from build123d import *

# Parameters (mm, degrees)
SKETCH1_R           = 3
BOSS_EXTRUDE1_DEPTH = 2.5
SKETCH2_R           = 1.5
BOSS_EXTRUDE2_DEPTH = 20
CHAMFER1_SIZE       = 2.5
CHAMFER1_SIZE_2     = 1.5
FILLET1_R           = 0.1
SKETCH3_W           = 1
SKETCH3_H           = 1
CUT_EXTRUDE2_DEPTH  = 1.5
CHAMFER7_SIZE       = 1.5
CHAMFER7_SIZE_2     = 0.3


with BuildPart() as part:
    # Sketch1 → Boss-Extrude1 (new body)
    with BuildSketch(Plane(origin=(0, 0, 0), x_dir=(1, 0, 0), z_dir=(0, 1, 0))):
        with Locations(Location((0, 0, 0), (0, 0, 270))):
            Circle(SKETCH1_R)
    extrude(amount=BOSS_EXTRUDE1_DEPTH)

    # Sketch2 → Boss-Extrude2 (add)
    with BuildSketch(Plane(origin=(0, 2.5, 0), x_dir=(1, 0, 0), z_dir=(0, 1, 0))):
        with Locations(Location((0, 0, 0), (0, 0, 270))):
            Circle(SKETCH2_R)
    extrude(amount=BOSS_EXTRUDE2_DEPTH)

    # Chamfer1
    # the kernel refuses this chamfer: 2.5, 1.5 mm, written as the material it takes off along each edge
    with BuildSketch(Plane(origin=(0, 2.5, 0), x_dir=(0, 0, 1), z_dir=(-1, 0, 0))) as chamfer1_piece_1_section:
        Polygon((3, -CHAMFER1_SIZE), (3 - CHAMFER1_SIZE_2, 0), (3, 0), align=None)
    chamfer1_piece_1 = revolve(axis=Axis((0, 2.5, 0), (0, 1, 0)), mode=Mode.PRIVATE)
    chamfer1_piece_1 = chamfer1_piece_1 - Plane(origin=(0, 2.5, 0), x_dir=(0, 0, 1), z_dir=(0, -1, 0)) * Cylinder(1.5, 12, mode=Mode.PRIVATE)
    add(chamfer1_piece_1, mode=Mode.SUBTRACT)

    # Fillet1
    fillet1_edges = [part.edges().sort_by_distance(p)[0] for p in [
        (0, 0, -3),
    ]]
    fillet(fillet1_edges, radius=FILLET1_R)

    # Sketch3 → Cut-Extrude2 (cut)
    with BuildSketch(Plane.XZ):
        with Locations((0, -1)):
            Rectangle(SKETCH3_W, SKETCH3_H)
        with Locations((-1, 0)):
            Rectangle(SKETCH3_W, SKETCH3_H)
        Rectangle(SKETCH3_W, SKETCH3_H)
        with Locations((0, 1)):
            Rectangle(SKETCH3_W, SKETCH3_H)
        with Locations((1, 0)):
            Rectangle(SKETCH3_W, SKETCH3_H)
    extrude(amount=-CUT_EXTRUDE2_DEPTH, mode=Mode.SUBTRACT)

    # Chamfer7
    # the kernel refuses this chamfer: 1.5, 0.3 mm, written as the material it adds along each edge
    with BuildSketch(Plane(origin=(-0.5, 1.5, -1.5), x_dir=(0, -1, 0), z_dir=(1, 0, 0)), Plane(origin=(0.5, 1.5, 1.5), x_dir=(0, -1, 0), z_dir=(-1, 0, 0)), Plane(origin=(1.5, 1.5, 0.5), x_dir=(0, -1, 0), z_dir=(-1, 0, 0)), Plane(origin=(-0.5, 1.5, 1.5), x_dir=(0, -1, 0), z_dir=(0, 0, -1)), Plane(origin=(-1.5, 1.5, 0.5), x_dir=(0, -1, 0), z_dir=(0, 0, -1)), Plane(origin=(1.5, 1.5, -0.5), x_dir=(0, -1, 0), z_dir=(0, 0, 1)), Plane(origin=(0.5, 1.5, -0.5), x_dir=(0, -1, 0), z_dir=(1, 0, 0)), Plane(origin=(-1.5, 1.5, -0.5), x_dir=(0, -1, 0), z_dir=(1, 0, 0)), Plane(origin=(-0.5, 1.5, -0.5), x_dir=(0, -1, 0), z_dir=(0, 0, -1))) as chamfer7_piece_1:
        Polygon((CHAMFER7_SIZE, 0), (0, -CHAMFER7_SIZE_2), (0, 0), align=None)
    extrude(amount=1)
    with BuildSketch(Plane(origin=(0.5, 1.5, 1.5), x_dir=(0, -1, 0), z_dir=(0, 0, -1)), Plane(origin=(-1.5, 1.5, 0.5), x_dir=(0, -1, 0), z_dir=(1, 0, 0)), Plane(origin=(0.5, 1.5, -0.5), x_dir=(0, -1, 0), z_dir=(0, 0, -1))) as chamfer7_piece_2:
        Polygon((CHAMFER7_SIZE, 0), (0, CHAMFER7_SIZE_2), (0, 0), align=None)
    extrude(amount=1)
    with BuildSketch(Plane(origin=(0.5, 1.5, 5.397198129), x_dir=(0, -1, 0), z_dir=(0, 0, -1))) as chamfer7_piece_3_section:
        Polygon((CHAMFER7_SIZE, 0), (0, CHAMFER7_SIZE_2), (0, 0), align=None)
    chamfer7_piece_3 = extrude(amount=8.794396259, mode=Mode.PRIVATE)
    chamfer7_piece_3 = split(chamfer7_piece_3, bisect_by=Plane(origin=(0.5, 1.5, -0.5), z_dir=(0, 0, -1)), keep=Keep.TOP, mode=Mode.PRIVATE)
    chamfer7_piece_3 = split(chamfer7_piece_3, bisect_by=Plane(origin=(0.5, 1.5, -1.5), z_dir=(0, 0, 1)), keep=Keep.TOP, mode=Mode.PRIVATE)
    add(chamfer7_piece_3)
    with BuildSketch(Plane(origin=(5.397198129, 1.5, 0.5), x_dir=(0, -1, 0), z_dir=(-1, 0, 0))) as chamfer7_piece_4_section:
        Polygon((CHAMFER7_SIZE, 0), (0, -CHAMFER7_SIZE_2), (0, 0), align=None)
    chamfer7_piece_4 = extrude(amount=8.794396259, mode=Mode.PRIVATE)
    chamfer7_piece_4 = split(chamfer7_piece_4, bisect_by=Plane(origin=(-1.5, 1.5, 0.5), z_dir=(1, 0, 0)), keep=Keep.TOP, mode=Mode.PRIVATE)
    chamfer7_piece_4 = split(chamfer7_piece_4, bisect_by=Plane(origin=(-0.5, 1.5, 0.5), z_dir=(-1, 0, 0)), keep=Keep.TOP, mode=Mode.PRIVATE)
    add(chamfer7_piece_4)
    with BuildSketch(Plane(origin=(-0.5, 1.5, 5.397198129), x_dir=(0, -1, 0), z_dir=(0, 0, -1))) as chamfer7_piece_5_section:
        Polygon((CHAMFER7_SIZE, 0), (0, -CHAMFER7_SIZE_2), (0, 0), align=None)
    chamfer7_piece_5 = extrude(amount=8.794396259, mode=Mode.PRIVATE)
    chamfer7_piece_5 = split(chamfer7_piece_5, bisect_by=Plane(origin=(-0.5, 1.5, -0.5), z_dir=(0, 0, -1)), keep=Keep.TOP, mode=Mode.PRIVATE)
    chamfer7_piece_5 = split(chamfer7_piece_5, bisect_by=Plane(origin=(-0.5, 1.5, -1.5), z_dir=(0, 0, 1)), keep=Keep.TOP, mode=Mode.PRIVATE)
    add(chamfer7_piece_5)
    with BuildSketch(Plane(origin=(-5.397198129, 1.5, 0.5), x_dir=(0, -1, 0), z_dir=(1, 0, 0))) as chamfer7_piece_6_section:
        Polygon((CHAMFER7_SIZE, 0), (0, CHAMFER7_SIZE_2), (0, 0), align=None)
    chamfer7_piece_6 = extrude(amount=8.794396259, mode=Mode.PRIVATE)
    chamfer7_piece_6 = split(chamfer7_piece_6, bisect_by=Plane(origin=(0.5, 1.5, 0.5), z_dir=(1, 0, 0)), keep=Keep.TOP, mode=Mode.PRIVATE)
    chamfer7_piece_6 = split(chamfer7_piece_6, bisect_by=Plane(origin=(1.5, 1.5, 0.5), z_dir=(-1, 0, 0)), keep=Keep.TOP, mode=Mode.PRIVATE)
    add(chamfer7_piece_6)
    with BuildSketch(Plane(origin=(-3.397198129, 1.5, -0.5), x_dir=(0, -1, 0), z_dir=(1, 0, 0))) as chamfer7_piece_7_section:
        Polygon((CHAMFER7_SIZE, 0), (0, -CHAMFER7_SIZE_2), (0, 0), align=None)
    chamfer7_piece_7 = extrude(amount=8.794396259, mode=Mode.PRIVATE)
    chamfer7_piece_7 = split(chamfer7_piece_7, bisect_by=Plane(origin=(-1.5, 1.5, -0.5), z_dir=(1, 0, 0)), keep=Keep.TOP, mode=Mode.PRIVATE)
    chamfer7_piece_7 = split(chamfer7_piece_7, bisect_by=Plane(origin=(-0.5, 1.5, -0.5), z_dir=(-1, 0, 0)), keep=Keep.TOP, mode=Mode.PRIVATE)
    add(chamfer7_piece_7)
    with BuildSketch(Plane(origin=(0.5, 1.5, 3.397198129), x_dir=(0, -1, 0), z_dir=(0, 0, -1))) as chamfer7_piece_8_section:
        Polygon((CHAMFER7_SIZE, 0), (0, CHAMFER7_SIZE_2), (0, 0), align=None)
    chamfer7_piece_8 = extrude(amount=8.794396259, mode=Mode.PRIVATE)
    chamfer7_piece_8 = split(chamfer7_piece_8, bisect_by=Plane(origin=(0.5, 1.5, 1.5), z_dir=(0, 0, -1)), keep=Keep.TOP, mode=Mode.PRIVATE)
    chamfer7_piece_8 = split(chamfer7_piece_8, bisect_by=Plane(origin=(0.5, 1.5, 0.5), z_dir=(0, 0, 1)), keep=Keep.TOP, mode=Mode.PRIVATE)
    add(chamfer7_piece_8)
    with BuildSketch(Plane(origin=(-5.397198129, 1.5, -0.5), x_dir=(0, -1, 0), z_dir=(1, 0, 0))) as chamfer7_piece_9_section:
        Polygon((CHAMFER7_SIZE, 0), (0, -CHAMFER7_SIZE_2), (0, 0), align=None)
    chamfer7_piece_9 = extrude(amount=8.794396259, mode=Mode.PRIVATE)
    chamfer7_piece_9 = split(chamfer7_piece_9, bisect_by=Plane(origin=(1.5, 1.5, -0.5), z_dir=(-1, 0, 0)), keep=Keep.TOP, mode=Mode.PRIVATE)
    chamfer7_piece_9 = split(chamfer7_piece_9, bisect_by=Plane(origin=(0.5, 1.5, -0.5), z_dir=(1, 0, 0)), keep=Keep.TOP, mode=Mode.PRIVATE)
    add(chamfer7_piece_9)
    with BuildSketch(Plane(origin=(-0.5, 1.5, 3.397198129), x_dir=(0, -1, 0), z_dir=(0, 0, -1))) as chamfer7_piece_10_section:
        Polygon((CHAMFER7_SIZE, 0), (0, -CHAMFER7_SIZE_2), (0, 0), align=None)
    chamfer7_piece_10 = extrude(amount=8.794396259, mode=Mode.PRIVATE)
    chamfer7_piece_10 = split(chamfer7_piece_10, bisect_by=Plane(origin=(-0.5, 1.5, 0.5), z_dir=(0, 0, 1)), keep=Keep.TOP, mode=Mode.PRIVATE)
    chamfer7_piece_10 = split(chamfer7_piece_10, bisect_by=Plane(origin=(-0.5, 1.5, 1.5), z_dir=(0, 0, -1)), keep=Keep.TOP, mode=Mode.PRIVATE)
    add(chamfer7_piece_10)
    with BuildSketch(Plane(origin=(0.5, 1.5, 1.5), x_dir=(0, -1, 0), z_dir=(0, 0, -1))) as chamfer7_piece_11a_section:
        Polygon((CHAMFER7_SIZE, 0), (0, CHAMFER7_SIZE_2), (0, 0), align=None)
    chamfer7_piece_11a = extrude(amount=4.897198129, mode=Mode.PRIVATE)
    chamfer7_piece_11a = split(chamfer7_piece_11a, bisect_by=Plane(origin=(0.5, 1.5, 0.5), z_dir=(0, 0, -1)), keep=Keep.TOP, mode=Mode.PRIVATE)
    chamfer7_piece_11a = split(chamfer7_piece_11a, bisect_by=Plane(origin=(0.5, 1.5, -0.5), z_dir=(0, 0, 1)), keep=Keep.TOP, mode=Mode.PRIVATE)
    with BuildSketch(Plane(origin=(1.5, 1.5, 0.5), x_dir=(0, -1, 0), z_dir=(-1, 0, 0))) as chamfer7_piece_11b_section:
        Polygon((CHAMFER7_SIZE, 0), (0, -CHAMFER7_SIZE_2), (0, 0), align=None)
    chamfer7_piece_11b = extrude(amount=4.897198129, mode=Mode.PRIVATE)
    chamfer7_piece_11b = split(chamfer7_piece_11b, bisect_by=Plane(origin=(-0.5, 1.5, 0.5), z_dir=(1, 0, 0)), keep=Keep.TOP, mode=Mode.PRIVATE)
    chamfer7_piece_11b = split(chamfer7_piece_11b, bisect_by=Plane(origin=(0.5, 1.5, 0.5), z_dir=(-1, 0, 0)), keep=Keep.TOP, mode=Mode.PRIVATE)
    chamfer7_piece_11 = chamfer7_piece_11a & chamfer7_piece_11b
    add(chamfer7_piece_11)
    with BuildSketch(Plane(origin=(-1.5, 1.5, 0.5), x_dir=(0, -1, 0), z_dir=(1, 0, 0))) as chamfer7_piece_12a_section:
        Polygon((CHAMFER7_SIZE, 0), (0, CHAMFER7_SIZE_2), (0, 0), align=None)
    chamfer7_piece_12a = extrude(amount=4.897198129, mode=Mode.PRIVATE)
    chamfer7_piece_12a = split(chamfer7_piece_12a, bisect_by=Plane(origin=(-0.5, 1.5, 0.5), z_dir=(1, 0, 0)), keep=Keep.TOP, mode=Mode.PRIVATE)
    chamfer7_piece_12a = split(chamfer7_piece_12a, bisect_by=Plane(origin=(0.5, 1.5, 0.5), z_dir=(-1, 0, 0)), keep=Keep.TOP, mode=Mode.PRIVATE)
    with BuildSketch(Plane(origin=(-0.5, 1.5, 1.5), x_dir=(0, -1, 0), z_dir=(0, 0, -1))) as chamfer7_piece_12b_section:
        Polygon((CHAMFER7_SIZE, 0), (0, -CHAMFER7_SIZE_2), (0, 0), align=None)
    chamfer7_piece_12b = extrude(amount=4.897198129, mode=Mode.PRIVATE)
    chamfer7_piece_12b = split(chamfer7_piece_12b, bisect_by=Plane(origin=(-0.5, 1.5, -0.5), z_dir=(0, 0, 1)), keep=Keep.TOP, mode=Mode.PRIVATE)
    chamfer7_piece_12b = split(chamfer7_piece_12b, bisect_by=Plane(origin=(-0.5, 1.5, 0.5), z_dir=(0, 0, -1)), keep=Keep.TOP, mode=Mode.PRIVATE)
    chamfer7_piece_12 = chamfer7_piece_12a & chamfer7_piece_12b
    add(chamfer7_piece_12)
    with BuildSketch(Plane(origin=(-3.397198129, 1.5, -0.5), x_dir=(0, -1, 0), z_dir=(1, 0, 0))) as chamfer7_piece_13a_section:
        Polygon((CHAMFER7_SIZE, 0), (0, -CHAMFER7_SIZE_2), (0, 0), align=None)
    chamfer7_piece_13a = extrude(amount=4.897198129, mode=Mode.PRIVATE)
    chamfer7_piece_13a = split(chamfer7_piece_13a, bisect_by=Plane(origin=(0.5, 1.5, -0.5), z_dir=(-1, 0, 0)), keep=Keep.TOP, mode=Mode.PRIVATE)
    chamfer7_piece_13a = split(chamfer7_piece_13a, bisect_by=Plane(origin=(-0.5, 1.5, -0.5), z_dir=(1, 0, 0)), keep=Keep.TOP, mode=Mode.PRIVATE)
    with BuildSketch(Plane(origin=(0.5, 1.5, 3.397198129), x_dir=(0, -1, 0), z_dir=(0, 0, -1))) as chamfer7_piece_13b_section:
        Polygon((CHAMFER7_SIZE, 0), (0, CHAMFER7_SIZE_2), (0, 0), align=None)
    chamfer7_piece_13b = extrude(amount=4.897198129, mode=Mode.PRIVATE)
    chamfer7_piece_13b = split(chamfer7_piece_13b, bisect_by=Plane(origin=(0.5, 1.5, 0.5), z_dir=(0, 0, -1)), keep=Keep.TOP, mode=Mode.PRIVATE)
    chamfer7_piece_13b = split(chamfer7_piece_13b, bisect_by=Plane(origin=(0.5, 1.5, -0.5), z_dir=(0, 0, 1)), keep=Keep.TOP, mode=Mode.PRIVATE)
    chamfer7_piece_13 = chamfer7_piece_13a & chamfer7_piece_13b
    add(chamfer7_piece_13)
    with BuildSketch(Plane(origin=(-1.5, 1.5, -0.5), x_dir=(0, -1, 0), z_dir=(1, 0, 0))) as chamfer7_piece_14a_section:
        Polygon((CHAMFER7_SIZE, 0), (0, -CHAMFER7_SIZE_2), (0, 0), align=None)
    chamfer7_piece_14a = extrude(amount=4.897198129, mode=Mode.PRIVATE)
    chamfer7_piece_14a = split(chamfer7_piece_14a, bisect_by=Plane(origin=(0.5, 1.5, -0.5), z_dir=(-1, 0, 0)), keep=Keep.TOP, mode=Mode.PRIVATE)
    chamfer7_piece_14a = split(chamfer7_piece_14a, bisect_by=Plane(origin=(-0.5, 1.5, -0.5), z_dir=(1, 0, 0)), keep=Keep.TOP, mode=Mode.PRIVATE)
    with BuildSketch(Plane(origin=(-0.5, 1.5, 3.397198129), x_dir=(0, -1, 0), z_dir=(0, 0, -1))) as chamfer7_piece_14b_section:
        Polygon((CHAMFER7_SIZE, 0), (0, -CHAMFER7_SIZE_2), (0, 0), align=None)
    chamfer7_piece_14b = extrude(amount=4.897198129, mode=Mode.PRIVATE)
    chamfer7_piece_14b = split(chamfer7_piece_14b, bisect_by=Plane(origin=(-0.5, 1.5, -0.5), z_dir=(0, 0, 1)), keep=Keep.TOP, mode=Mode.PRIVATE)
    chamfer7_piece_14b = split(chamfer7_piece_14b, bisect_by=Plane(origin=(-0.5, 1.5, 0.5), z_dir=(0, 0, -1)), keep=Keep.TOP, mode=Mode.PRIVATE)
    chamfer7_piece_14 = chamfer7_piece_14a & chamfer7_piece_14b
    add(chamfer7_piece_14)


solid = part.part
For this review, take the finished solid that the model builds, in its own axes (mm). A direction names the side the tool comes from. Give positions to 0.01 mm unless a question says otherwise; leave off trailing zeros. Loops run counter-clockwise (first coordinate to the right, second up) from the corner with the lowest first, then second, coordinate; pieces in that order, holes last. Notation, with made-up numbers: M 9.5,-28 L 38.5,-28 A22 ccw 38.5,-22 Z; hole C 27,69 d5. An arc over 180 degrees is marked long. Put each result on its own line as item: value. Start each with the question number.
(1) The part is to be moulded in two halves that separate along X. For faces 1 (the flat face through (-1, 0, 1)), 2 (the cylindrical face through (0.45, 12.36, 1.43)), 3 (the flat face through (0.86, 0.74, 0.35)), say which applies: +X half, -X half, draft (parallel to the pull), parting line (faces both ways), or undercut.
(2) Add section D-D, the plane y = 11.5. Write out the cut boundary in (x, z), then the cut area to 3 significant figures.
(3) For pin 1 (2 mm diameter, centred on x = -2, y = 3, fed in from -Z); pin 2 (1 mm diameter, centred on x = 0.5, y = 8, fed in from +Z); pin 3 (2 mm diameter, centred on y = 7, z = 1.5, fed in from +X), all flat-tipped, find the tip position at first contact; note any pin that passes through.
(4) Add section B-B, the plane z = 0. Write out the cut boundary in (x, y), then the cut area to 3 significant figures.
(5) Machinability: for faces 4 (the flat face through (0, 1.5, 0)), 5 (the flat face through (0, 22.5, 0)), which of the approach directions +Z, -Z, +X, -X, +Y, -Y give a long, thin tool a straight path to every point of the face, cutting with its end or side? Answer none if there is none.
(6) Add section A-A, the plane x = 0. Write out the cut boundary in (y, z), then the cut area to 3 significant figures.
(7) Wall thickness on L1, parallel to X at y = 21.5, z = -0.1; L2, parallel to Y at x = 0.3, z = 2.3: over which ranges is each line inside the solid? List them lowest first.
(8) Add section C-C, the plane y = 2. Write out the cut boundary in (x, z), then the cut area to 3 significant figures.
Result:
1. face 1: draft
1. face 2: parting line
1. face 3: undercut
2. outline: C 0,0 d3
2. area: 7.07 mm^2
3. pin 1: stops at z = -1.12
3. pin 2: stops at z = 1.5
3. pin 3: stops at x = 1.41
4. outline: M -2.91,0.15 A0.1 ccw -2.82,0 L -1.5,0 L -1.2,1.5 L 1.2,1.5 L 1.5,0 L 2.82,0 A0.1 ccw 2.91,0.15 L 1.5,2.5 L 1.5,22.5 L -1.5,22.5 L -1.5,2.5 Z
4. area: 67.2 mm^2
5. face 4: -Y
5. face 5: +Z, -Z, +X, -X, +Y
6. outline: M 0,-2.82 A0.1 ccw 0.15,-2.91 L 2.5,-1.5 L 22.5,-1.5 L 22.5,1.5 L 2.5,1.5 L 0.15,2.91 A0.1 ccw 0,2.82 L 0,1.5 L 1.5,1.2 L 1.5,-1.2 L 0,-1.5 Z
6. area: 67.2 mm^2
7. L1: x = -1.5 to 1.5
7. L2: y = 0 to 1.13
8. outline: C 0,0 d3.6
8. area: 10.2 mm^2
